Design review of the part built by this model. Coordinates are the model's own, in mm. A direction names the side the tool comes from. Give positions to 0.01 mm unless a question says otherwise; leave off trailing zeros. Loops run counter-clockwise (first coordinate to the right, second up) from the corner with the lowest first, then second, coordinate; pieces in that order, holes last. Notation, with made-up numbers: (59, -36.5) -> (81, -36.5) arc R19 ccw to (81, -25.5) -> close; hole circle Ø6 at (72.25, 51.25). An arc over 180 degrees is marked (long way). Answer as CSV lines item,"result".
from build123d import *

# Parameters (mm, degrees)
EXTRUDE_1_DEPTH     = 5
CUT_EXTRUDE_1_DEPTH = 1.5
CUT_EXTRUDE_2_DEPTH = 2.5
SKETCH_4_R          = 1.25
CUT_EXTRUDE_3_DEPTH = 5
SKETCH_5_R          = 2.85
CUT_EXTRUDE_4_DEPTH = 3.5
SKETCH_6_R          = 1.25
CUT_EXTRUDE_5_DEPTH = 5
SKETCH_7_R          = 2.85
CUT_EXTRUDE_6_DEPTH = 3.5
SKETCH_8_W          = 2
SKETCH_8_H          = 130
CUT_EXTRUDE_8_DEPTH = 1


with BuildPart() as part:
    # 草图1 → 凸台-拉伸1 (new body)
    with BuildSketch(Plane(origin=(0, 0, 0), x_dir=(1, 0, 0), z_dir=(0, 1, 0))):
        with BuildLine():
            Line((-120, 75), (120, 75))
            ThreePointArc((120, 75), (123.535533906, 73.535533906), (125, 70))
            Line((125, 70), (125, -70))
            ThreePointArc((125, -70), (123.535533906, -73.535533906), (120, -75))
            Line((120, -75), (-120, -75))
            ThreePointArc((-120, -75), (-123.535533906, -73.535533906), (-125, -70))
            Line((-125, -70), (-125, 70))
            ThreePointArc((-125, 70), (-123.535533906, 73.535533906), (-120, 75))
        make_face()
    extrude(amount=EXTRUDE_1_DEPTH)

    # 草图2 → 切除-拉伸1 (cut)
    with BuildSketch(Plane(origin=(0, 5, 0), x_dir=(1, 0, 0), z_dir=(0, 1, 0))):
        with BuildLine():
            Line((-125, 60), (-120, 60))
            ThreePointArc((-120, 60), (-116.464466094, 58.535533906), (-115, 55))
            Line((-115, 55), (-115, -55))
            ThreePointArc((-115, -55), (-116.464466094, -58.535533906), (-120, -60))
            Line((-120, -60), (-125, -60))
            Line((-125, -60), (-125, 60))
        make_face()
        with BuildLine():
            Line((115, 55), (115, -55))
            ThreePointArc((115, -55), (116.464466094, -58.535533906), (120, -60))
            Line((120, -60), (125, -60))
            Line((125, -60), (125, 60))
            Line((125, 60), (120, 60))
            ThreePointArc((120, 60), (116.464466094, 58.535533906), (115, 55))
        make_face()
    extrude(amount=-CUT_EXTRUDE_1_DEPTH, mode=Mode.SUBTRACT)

    # 草图3 → 切除-拉伸2 (cut)
    with BuildSketch(Plane(origin=(0, 5, 0), x_dir=(1, 0, 0), z_dir=(0, 1, 0))):
        with BuildLine():
            Line((-100, 67), (100, 67))
            ThreePointArc((100, 67), (104.949747468, 64.949747468), (107, 60))
            Line((107, 60), (107, -60))
            ThreePointArc((107, -60), (104.949747468, -64.949747468), (100, -67))
            Line((100, -67), (-100, -67))
            ThreePointArc((-100, -67), (-104.949747468, -64.949747468), (-107, -60))
            Line((-107, -60), (-107, 60))
            ThreePointArc((-107, 60), (-104.949747468, 64.949747468), (-100, 67))
        make_face()
        with BuildLine():
            Line((-100, 65), (100, 65))
            ThreePointArc((100, 65), (103.535533906, 63.535533906), (105, 60))
            Line((105, 60), (105, -60))
            ThreePointArc((105, -60), (103.535533906, -63.535533906), (100, -65))
            Line((100, -65), (-100, -65))
            ThreePointArc((-100, -65), (-103.535533906, -63.535533906), (-105, -60))
            Line((-105, -60), (-105, 60))
            ThreePointArc((-105, 60), (-103.535533906, 63.535533906), (-100, 65))
        make_face(mode=Mode.SUBTRACT)
    extrude(amount=-CUT_EXTRUDE_2_DEPTH, mode=Mode.SUBTRACT)

    # 草图4 → 切除-拉伸3 (cut)
    with BuildSketch(Plane.XZ):
        with Locations(Location((-120, 70, 0), (0, 0, 270))):
            Circle(SKETCH_4_R)
        with Locations(Location((-120, -70, 0), (0, 0, 270))):
            Circle(SKETCH_4_R)
        with Locations(Location((120, -70, 0), (0, 0, 270))):
            Circle(SKETCH_4_R)
        with Locations(Location((120, 70, 0), (0, 0, 270))):
            Circle(SKETCH_4_R)
    extrude(amount=-CUT_EXTRUDE_3_DEPTH, mode=Mode.SUBTRACT)

    # 草图5 → 切除-拉伸4 (cut)
    with BuildSketch(Plane.XZ):
        with Locations(Location((-120, 70, 0), (0, 0, 270))):
            Circle(SKETCH_5_R)
        with Locations(Location((-120, -70, 0), (0, 0, 270))):
            Circle(SKETCH_5_R)
        with Locations(Location((120, -70, 0), (0, 0, 270))):
            Circle(SKETCH_5_R)
        with Locations(Location((120, 70, 0), (0, 0, 270))):
            Circle(SKETCH_5_R)
    extrude(amount=-CUT_EXTRUDE_4_DEPTH, mode=Mode.SUBTRACT)

    # 草图6 → 切除-拉伸5 (cut)
    with BuildSketch(Plane(origin=(0, 5, 0), x_dir=(1, 0, 0), z_dir=(0, 1, 0))):
        with Locations(Location((0, 71, 0), (0, 0, 270))):
            Circle(SKETCH_6_R)
        with Locations(Location((-60.164669271, 71, 0), (0, 0, 270))):
            Circle(SKETCH_6_R)
        with Locations(Location((60.164669271, 71, 0), (0, 0, 90))):
            Circle(SKETCH_6_R)
        with Locations(Location((60.164669271, -71, 0), (0, 0, 270))):
            Circle(SKETCH_6_R)
        with Locations(Location((-60.164669271, -71, 0), (0, 0, 90))):
            Circle(SKETCH_6_R)
        with Locations(Location((0, -71, 0), (0, 0, 90))):
            Circle(SKETCH_6_R)
    extrude(amount=-CUT_EXTRUDE_5_DEPTH, mode=Mode.SUBTRACT)

    # 草图7 → 切除-拉伸6 (cut)
    with BuildSketch(Plane.XZ):
        with Locations(Location((-60.164669271, 71, 0), (0, 0, 270))):
            Circle(SKETCH_7_R)
        with Locations(Location((0, 71, 0), (0, 0, 270))):
            Circle(SKETCH_7_R)
        with Locations(Location((60.164669271, 71, 0), (0, 0, 270))):
            Circle(SKETCH_7_R)
        with Locations(Location((60.164669271, -71, 0), (0, 0, 90))):
            Circle(SKETCH_7_R)
        with Locations(Location((0, -71, 0), (0, 0, 90))):
            Circle(SKETCH_7_R)
        with Locations(Location((-60.164669271, -71, 0), (0, 0, 90))):
            Circle(SKETCH_7_R)
    extrude(amount=-CUT_EXTRUDE_6_DEPTH, mode=Mode.SUBTRACT)

    # 草图8 → 切除-拉伸8 (cut)
    with BuildSketch(Plane(origin=(0, 5, 0), x_dir=(1, 0, 0), z_dir=(0, 1, 0))):
        Rectangle(SKETCH_8_W, SKETCH_8_H)
    extrude(amount=-CUT_EXTRUDE_8_DEPTH, mode=Mode.SUBTRACT)


solid = part.part
Q1. For faces 4 (the flat face through (-1, 3.5, 70)), 5 (the cylindrical face through (105, 3.8, 64.9)), 6 (the cylindrical face through (123, 2, -74)), list the 3-axis set-ups (+Z, -Z, +X, -X, +Y, -Y) from which the entire face can be reached by the end or side of a thin tool; tool diameter is ignored.
Filled sheet:
face 4,"-Y"
face 5,"+Y"
face 6,"-Z, +X, +Y, -Y"
Q2. To check wall thickness, follow probe 1 along Z at (x, y) = (-51.5, 3.3); probe 2 along Z at (x, y) = (-120, 4.25); probe 3 along X at (y, z) = (4.7, -25.5). State the ranges of each line that lie inside material, in increasing order. Write a range as from..to.
Filled sheet:
probe 1,"z = -75..-67, -65..65, 67..75"
probe 2,"z = -75..-71.25, -68.75..-60, 60..68.75, 71.25..75"
probe 3,"x = -115..-107, -105..-1, 1..105, 107..115"
Q3. The part is to be moulded in two halves that separate along Z. For faces 1 (the cylindrical face through (61.26, 1.73, -68.37)), 2 (the flat face through (2, 0, -1)), 3 (the flat face through (-2, 2, -75)), say which applies: pulls with the +Z half, pulls with the -Z half, needs draft (parallel to the pull), parting line crosses it, or undercut.
Filled sheet:
face 1,"undercut"
face 2,"needs draft"
face 3,"pulls with the -Z half"
Q4. We need section A-A, the plane z = -16. State the section outline as (x, y) points, and give its area (3 significant figures).
Filled sheet:
outline,"(-125, 0) -> (125, 0) -> (125, 3.5) -> (115, 3.5) -> (115, 5) -> (107, 5) -> (107, 2.5) -> (105, 2.5) -> (105, 5) -> (1, 5) -> (1, 4) -> (-1, 4) -> (-1, 5) -> (-105, 5) -> (-105, 2.5) -> (-107, 2.5) -> (-107, 5) -> (-115, 5) -> (-115, 3.5) -> (-125, 3.5) -> close"
area,"1,210 mm^2"
Q5. Clearance check with flat-ended pins moving along their axes: pin 1 Ø1.7 at (x, z) = (59, -71) entering from -Y; pin 2 Ø2 at (x, z) = (60.16, 71) entering from -Y; pin 3 Ø1 at (x, z) = (0, 0.5) entering from +Y; pin 4 Ø0.8 at (y, z) = (4.5, -11.5) entering from -X. State where each tip first meets the part, or that it passes through.
Filled sheet:
pin 1,"stops at y = 3.5"
pin 2,"passes through"
pin 3,"stops at y = 4"
pin 4,"stops at x = -115"
